from build123d import *

# Parameters (mm, degrees)
BOSS_EXTRUDE1_DEPTH      = 3
BOSS_EXTRUDE1_DEPTH_BACK = 3
M3_CLEARANCE_HOLE1_D     = 3.2
M3_CLEARANCE_HOLE1_DEPTH = 3.947545897
M3_CLEARANCE_HOLE2_D     = 3.2
M3_CLEARANCE_HOLE2_DEPTH = 3.330741851


with BuildPart() as part:
    # Sketch1 → Boss-Extrude1 (new body, two sides)
    with BuildSketch(Plane.XY) as boss_extrude1_sk:
        Polygon((-7.378385455, 23.969381317), (22.968373629, 23.969381317), (22.968373629, -8.104429097), (26.29911548, -8.104429097), (26.29911548, 27.916927214), (-7.378385455, 27.916927214), align=None)
    extrude(amount=BOSS_EXTRUDE1_DEPTH)
    extrude(boss_extrude1_sk.sketch, amount=-BOSS_EXTRUDE1_DEPTH_BACK)

    # M3 Clearance Hole1
    with Locations(Plane(origin=(0, 27.916927214, 0), x_dir=(1, 0, 0), z_dir=(0, 1, 0))):
        with Locations((0, 0)):
            Hole(M3_CLEARANCE_HOLE1_D / 2, depth=M3_CLEARANCE_HOLE1_DEPTH)

    # M3 Clearance Hole2
    with Locations(Plane(origin=(26.29911548, 0, 0), x_dir=(0, 0, -1), z_dir=(1, 0, 0))):
        with Locations((0, 0)):
            Hole(M3_CLEARANCE_HOLE2_D / 2, depth=M3_CLEARANCE_HOLE2_DEPTH)


solid = part.part
Verification items for the finished model (mm, model axes). A direction names the side the tool comes from. Round coordinates to 2 decimals unless told otherwise and drop trailing zeros. Loops run counter-clockwise (first coordinate to the right, second up) from the corner with the lowest first, then second, coordinate; pieces in that order, holes last. Notation, with made-up numbers: M 27.25,47.5 L 66.25,47.5 A21 cw 66.25,77.5 Z; hole C -5,75 d3. An arc over 180 degrees is marked long. Write each question's results on one line, items separated by ' | '.
1) Mould release check, pull along Y, two halves, no side actions. Record for faces 3 (the flat face through (16, 25, 3)), 4 (the cylindrical face through (24.61, -0.97, -1.27)), 5 (the flat face through (10, 27.917, 0)), 6 (the flat face through (25, -8.104, 0)): released by +Y, released by -Y, zero draft, split by the parting line, or undercut.
Checks:
face 3: zero draft | face 4: undercut | face 5: released by +Y | face 6: released by -Y
2) Access from +Z, -Z, +X, -X, +Y, -Y to the whole of each face (thin tool, end or side, straight path). Record for faces 1 (the cylindrical face through (1.27, 25.92, 0.97)), 2 (the flat face through (22.968, 8, 0)).
Checks:
face 1: +Y, -Y | face 2: +Z, -Z, -X, -Y
3) Section check B-B on x = 0. Record the boundary of the cut face in (y, z), then the cut area to 3 significant figures.
Checks:
outline: M 23.97,-3 L 27.92,-3 L 27.92,-1.6 L 23.97,-1.6 Z; M 23.97,1.6 L 27.92,1.6 L 27.92,3 L 23.97,3 Z | area: 11.1 mm2
4) Gauge pin test, flat end, axial feed: P1, Ø2, axis at x = 11.5, z = 1.5, coming from the -Y side. Record the tip position at first contact, or that the pin passes through.
Checks:
P1: stops at y = 23.97
5) Section check C-C on y = 0. Record the boundary of the cut face in (x, z).
Checks:
outline: M 22.97,-3 L 26.3,-3 L 26.3,-1.6 L 22.97,-1.6 Z; M 22.97,1.6 L 26.3,1.6 L 26.3,3 L 22.97,3 Z
6) Section check A-A on z = 0. Record the boundary of the cut face in (x, y), then the cut area to 3 significant figures.
Checks:
outline: M -7.38,23.97 L -1.6,23.97 L -1.6,27.92 L -7.38,27.92 Z; M 1.6,23.97 L 22.97,23.97 L 22.97,1.6 L 26.3,1.6 L 26.3,27.92 L 1.6,27.92 Z; M 22.97,-8.1 L 26.3,-8.1 L 26.3,-1.6 L 22.97,-1.6 Z | area: 216 mm2
7) Scan lines: L1, parallel to Y at x = 24.55, z = 0; L2, parallel to Z at x = 0, y = 26.05; L3, parallel to X at y = 6, z = -1.3. Record each from-to range of solid material in increasing order. Write a range as from..to.
Checks:
L1: y = -8.1..-1.6, 1.6..27.92 | L2: z = -3..-1.6, 1.6..3 | L3: x = 22.97..26.3
8) Section check D-D on x = 17.5. Record the boundary of the cut face in (y, z), then the cut area to 3 significant figures.
Checks:
outline: M 23.97,-3 L 27.92,-3 L 27.92,3 L 23.97,3 Z | area: 23.7 mm2
